from build123d import *

# Parameters (mm, degrees)
F1_DEPTH  = 2
F3_DEPTH  = 12
F5_DEPTH  = 10
F6_R      = 2
F7_W      = 10.4
F7_H      = 2.6
F8_DEPTH  = 10
F9_W      = 5
F9_H      = 6
F9_R      = 1.6
F10_DEPTH = 5
F11_R     = 1.6
F12_DEPTH = 5
F13_R     = 1.6
F14_DEPTH = 5
F15_R     = 2
F16_R     = 3.7
F17_DEPTH = 2.6
F18_R     = 3.7
F19_DEPTH = 2.6
F20_R     = 3.7
F21_DEPTH = 2.6
F22_R     = 2
F22_R_2   = 0.9
F23_DEPTH = 8


# Not quite as in the source:
# - a feature names something its author has since deleted; it is built from what else it names


with BuildPart() as f1:
    # F0 (on Front) → F1 (new body)
    with BuildSketch(Plane.XZ):
        Polygon((47.128, -40.814), (0, 40.8140904591), (-47.128, -40.814), align=None)
        Polygon((-29.8074919243, -30.814), (0, 20.8140904591), (29.8074919243, -30.814), align=None, mode=Mode.SUBTRACT)
    extrude(amount=F1_DEPTH)

    # F2 (on face) → F3 (join)
    with BuildSketch(Plane.XZ.offset(2)):
        Polygon((0, 40.8140904591), (-47.128, -40.814), (47.128, -40.814), align=None)
        Polygon((43.6638983849, -38.814), (-43.6638983849, -38.814), (0, 36.8140904591), align=None, mode=Mode.SUBTRACT)
    extrude(amount=F3_DEPTH)

    # F4 (on face) → F5 (join)
    with BuildSketch(Plane.XZ.offset(2)):
        Polygon((33.2715935394, -32.814), (0, 24.8140904591), (-33.2715935394, -32.814), align=None)
        Polygon((-29.8074919243, -30.814), (0, 20.8140904591), (29.8074919243, -30.814), align=None, mode=Mode.SUBTRACT)
    extrude(amount=F5_DEPTH)

    # F6
    f6_edges = [f1.edges().sort_by_distance(p)[0] for p in [
        (47.128, -7, -40.814),
        (-47.128, -7, -40.814),
        (0, -7, 40.81409),
        (-29.807492, -6, -30.814),
        (-43.663898, -8, -38.814),
        (0, -7, 24.81409),
        (0, -6, 20.81409),
        (0, -8, 36.81409),
        (33.271594, -7, -32.814),
        (-33.271594, -7, -32.814),
        (29.807492, -6, -30.814),
        (43.663898, -8, -38.814),
    ]]
    fillet(f6_edges, radius=F6_R)

    # F7 (on face) → F8 (join)
    with BuildSketch(Plane.XZ.offset(2)):
        Polygon((-31.9803847577, -23.7775607869), (-34.2320508076, -22.4775607869), (-39.4320508076, -31.4842249862), (-37.1803847577, -32.7842249862), align=None)
        Polygon((-9.4320508076, 20.4772992408), (-7.1803847577, 19.1772992408), (-1.9803847577, 28.1839634402), (-4.2320508076, 29.4839634402), align=None)
        Polygon((9.4320508076, 20.4772992408), (4.2320508076, 29.4839634402), (1.9803847577, 28.1839634402), (7.1803847577, 19.1772992408), align=None)
        Polygon((39.4320508076, -31.4842249862), (34.2320508076, -22.4775607869), (31.9803847577, -23.7775607869), (37.1803847577, -32.7842249862), align=None)
        with Locations((29.9997967697, -37.514)):
            Rectangle(F7_W, F7_H)
        with Locations((-30.0002032303, -37.514)):
            Rectangle(F7_W, F7_H)
    extrude(amount=F8_DEPTH)

    # F9 (on face) → F10 (cut)
    with BuildSketch(Plane(origin=(0, 0, -40.814), x_dir=(1, 0, 0), z_dir=(0, 0, -1))):
        with Locations((0, 11)):
            Rectangle(F9_W, F9_H)
        with Locations((-30.0002032303, 7)):
            Circle(F9_R)
        with Locations((29.9997967697, 7)):
            Circle(F9_R)
    extrude(amount=-F10_DEPTH, mode=Mode.SUBTRACT)

    # F11 (on face) → F12 (cut)
    with BuildSketch(Plane(origin=(17.673019585, 0, 10.2035226148), x_dir=(0, 1, 0), z_dir=(0.8660254038, 0, 0.5))):
        with Locations((-7, 18.2178359397)):
            Circle(F11_R)
        with Locations((-7, -41.7821640603)):
            Circle(F11_R)
    extrude(amount=-F12_DEPTH, mode=Mode.SUBTRACT)

    # F13 (on face) → F14 (cut)
    with BuildSketch(Plane(origin=(-17.673019585, 0, 10.2035226148), x_dir=(0, -1, 0), z_dir=(-0.8660254038, 0, 0.5))):
        with Locations((7, 18.2178359397)):
            Circle(F13_R)
        with Locations((7, -41.7821640603)):
            Circle(F13_R)
    extrude(amount=-F14_DEPTH, mode=Mode.SUBTRACT)

    # F15
    f15_edges = [f1.edges().sort_by_distance(p)[0] for p in [
        (-2.5, -8, -39.814),
        (2.5, -8, -39.814),
    ]]
    fillet(f15_edges, radius=F15_R)

    # F16 (on face) → F17 (cut)
    with BuildSketch(Plane.XY.offset(-36.214)):
        with Locations((29.9997967697, -7)):
            Circle(F16_R)
        with Locations((-30.0002032303, -7)):
            Circle(F16_R)
    extrude(amount=-F17_DEPTH, mode=Mode.SUBTRACT)

    # F18 (on face) → F19 (cut)
    with BuildSketch(Plane(origin=(13.6893027276, 0, 7.9035226148), x_dir=(0, -1, 0), z_dir=(-0.8660254038, 0, -0.5))):
        with Locations((7, -41.7821640603)):
            Circle(F18_R)
        with Locations((7, 18.2178359397)):
            Circle(F18_R)
    extrude(amount=-F19_DEPTH, mode=Mode.SUBTRACT)

    # F20 (on face) → F21 (cut)
    with BuildSketch(Plane(origin=(-13.6893027276, 0, 7.9035226148), x_dir=(0, 1, 0), z_dir=(0.8660254038, 0, -0.5))):
        with Locations((-7, -41.7821640603)):
            Circle(F20_R)
        with Locations((-7, 18.2178359397)):
            Circle(F20_R)
    extrude(amount=-F21_DEPTH, mode=Mode.SUBTRACT)

    # F22 (on face) → F23 (join)
    with BuildSketch(Plane.XZ.offset(2)):
        with Locations((0, 26.8140904591)):
            Circle(F22_R)
        with Locations((0, 26.8140904591)):
            Circle(F22_R_2, mode=Mode.SUBTRACT)
        with Locations((35.003644347, -33.814)):
            Circle(F22_R)
        with Locations((35.003644347, -33.814)):
            Circle(F22_R_2, mode=Mode.SUBTRACT)
        with Locations((-35.003644347, -33.814)):
            Circle(F22_R)
        with Locations((-35.003644347, -33.814)):
            Circle(F22_R_2, mode=Mode.SUBTRACT)
    extrude(amount=F23_DEPTH)


solid = f1.part
Source: CAD feature listing. Evaluate the final solid. Frame: model axes, mm. A direction names the side the tool comes from. Coordinates: 2 decimals unless noted, no trailing zeros. Order: outer loops, then holes, each group sorted by start corner. A loop starts at its lowest first (then second) coordinate and runs counter-clockwise, first axis right, second up.
Item 1: Cut plane B-B (y = -7). Count the separate pieces of the cut face and the enclosed holes in it, plus the area to 3 significant figures.
Output values:
separate pieces: 10
enclosed holes: 4
area: 962 mm2
Item 2: First-contact query: P1, Ø0.5, axis at x = 34.5, z = -33.5, coming from the -Y side; P2, Ø2, axis at x = 35, z = -33.81, coming from the -Y side; P3, Ø1, axis at y = -4, z = 0, coming from the -X side. Flat tips, straight axial feed; report the tip coordinate or a pass-through.
Output values:
P1: stops at y = -2
P2: stops at y = -10
P3: stops at x = -23.85
Item 3: Material intervals for line 1 (X direction, y = -2.25, z = -11.5); line 2 (Z direction, x = 4, y = -11.25); line 3 (X direction, y = -7, z = -10), sorted ascending.
Output values:
line 1: x = -30.2 to -27.89, -20.97 to -18.66, 18.66 to 20.97, 27.89 to 30.2
line 2: z = -40.81 to -38.81, -32.81 to -30.81, 13.89 to 17.89, 24.69 to 29.35, 29.89 to 33.89
line 3: x = -29.34 to -27.03, -20.1 to -17.79, 17.79 to 20.1, 27.03 to 29.34
Item 4: Set-up query: faces 1 (the face through (14.72, -5.92, -4.68)), 2 (the face through (-29, -9, -38.814)), 3 (the face through (-16, -2, -2)). Return all of +Z, -Z, +X, -X, +Y, -Y with unobstructed straight access to the full face (end or side cutting, diameter ignored); none if empty.
Output values:
face 1: +Y, -Y
face 2: none
face 3: -Y
Item 5: Cut plane A-A (z = -14). Return loops of the section in (x, y), plus the area to 3 significant figures.
Output values:
outline: (-31.65, -14) - (-29.34, -14) - (-29.34, -2) - (-22.41, -2) - (-22.41, -12) - (-20.1, -12) - (-20.1, 0) - (-31.65, 0) - close; (20.1, -12) - (22.41, -12) - (22.41, -2) - (29.34, -2) - (29.34, -14) - (31.65, -14) - (31.65, 0) - (20.1, 0) - close
area: 148 mm2
